The drawing under review shows one solid part. Ordinate dimensions are in mm from its lowest x, y, z. A direction names the side the tool comes from. Round coordinates to 2 decimals unless told otherwise and drop trailing zeros. Order: outer loops, then holes, each group sorted by start corner. A loop starts at its lowest first (then second) coordinate and runs counter-clockwise, first axis right, second up.
1) Clearance check with flat-ended pins moving along their axes: P1, Ø1.2, axis at x = 2.5, y = 4.5, coming from the -Z side; P2, Ø2, axis at x = 7, z = 10.5, coming from the -Y side; P3, Ø2.5, axis at x = 11, z = 22, coming from the +Y side; P4, Ø4, axis at x = 9.5, z = 37, coming from the -Y side. State where each tip first meets the part, or that it passes through.
2) Machinability: for the marked faces 1 and 2, which of the approach directions +Z, -Z, +X, -X, +Y, -Y give a long, thin tool a straight path to every point of the face, cutting with its end or side? Answer none if there is none.
3) To check wall thickness, follow L1, parallel to Z at x = 11, y = 2.5; L2, parallel to Z at x = 11, y = 11.5; L3, parallel to X at y = 1.5, z = 15.5. State the ranges of each line that lie inside material, in increasing order.
4) Consider section D-D (y = 11.25). Give the boundary of the cut face in (x, z), then the cut area to 3 significant figures.
5) Consider section A-A (z = 22). Give the boundary of the cut face in (x, y).
6) Consider section B-B (x = 11). Give the boundary of the cut face in (y, z).
7) Consider section C-C (y = 3). Give the boundary of the cut face in (x, z), then the cut area to 3 significant figures.
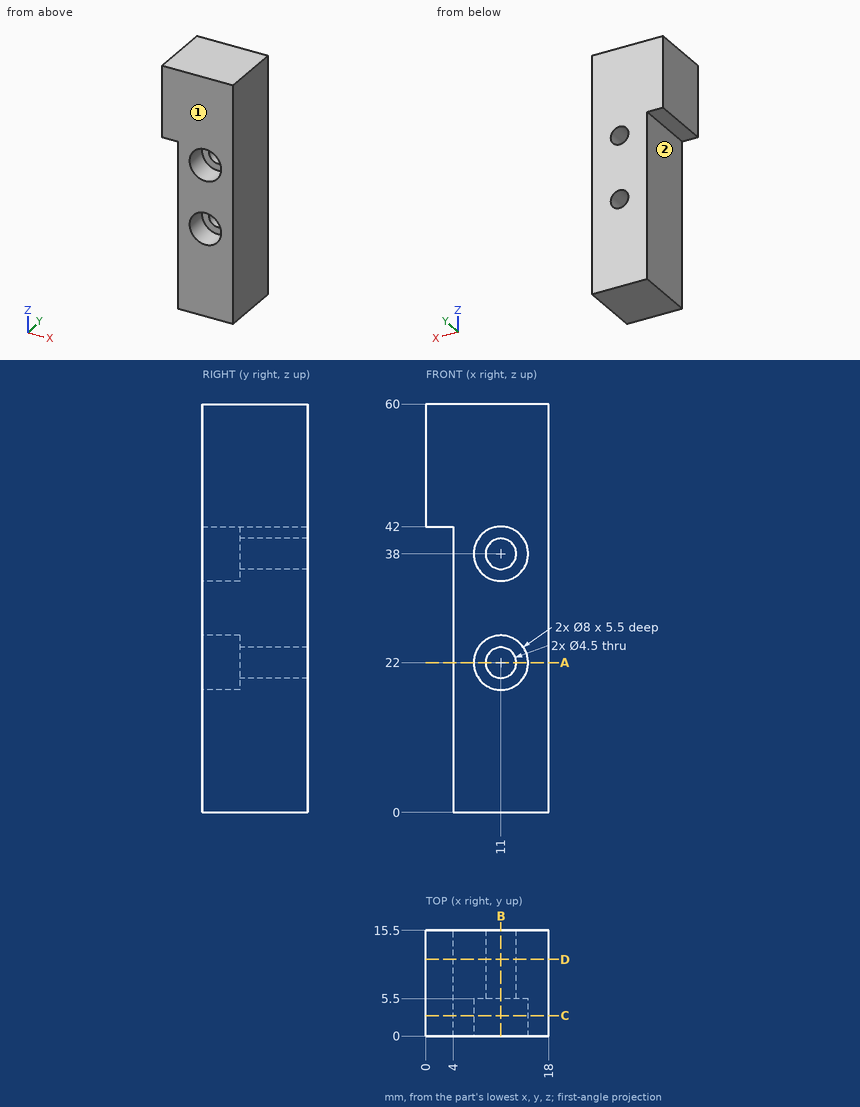
Answer below:
1. P1: stops at z = 42
1. P2: stops at y = 0
1. P3: passes through
1. P4: stops at y = 5.5
2. face 1: +Z, -Z, +X, -X, -Y
2. face 2: -Z, -X, +Y, -Y
3. L1: z = 0 to 18, 26 to 34, 42 to 60
3. L2: z = 0 to 19.75, 24.25 to 35.75, 40.25 to 60
3. L3: x = 4 to 18
4. outline: (0, 42) - (4, 42) - (4, 0) - (18, 0) - (18, 60) - (0, 60) - close; hole circle Ø4.5 at (11, 22); hole circle Ø4.5 at (11, 38)
4. area: 880 mm2
5. outline: (4, 0) - (7, 0) - (7, 5.5) - (8.75, 5.5) - (8.75, 15.5) - (4, 15.5) - close; (13.25, 5.5) - (15, 5.5) - (15, 0) - (18, 0) - (18, 15.5) - (13.25, 15.5) - close
6. outline: (0, 0) - (15.5, 0) - (15.5, 19.75) - (5.5, 19.75) - (5.5, 18) - (0, 18) - close; (0, 26) - (5.5, 26) - (5.5, 24.25) - (15.5, 24.25) - (15.5, 35.75) - (5.5, 35.75) - (5.5, 34) - (0, 34) - close; (0, 42) - (5.5, 42) - (5.5, 40.25) - (15.5, 40.25) - (15.5, 60) - (0, 60) - close
7. outline: (0, 42) - (4, 42) - (4, 0) - (18, 0) - (18, 60) - (0, 60) - close; hole circle Ø8 at (11, 22); hole circle Ø8 at (11, 38)
7. area: 811 mm2
